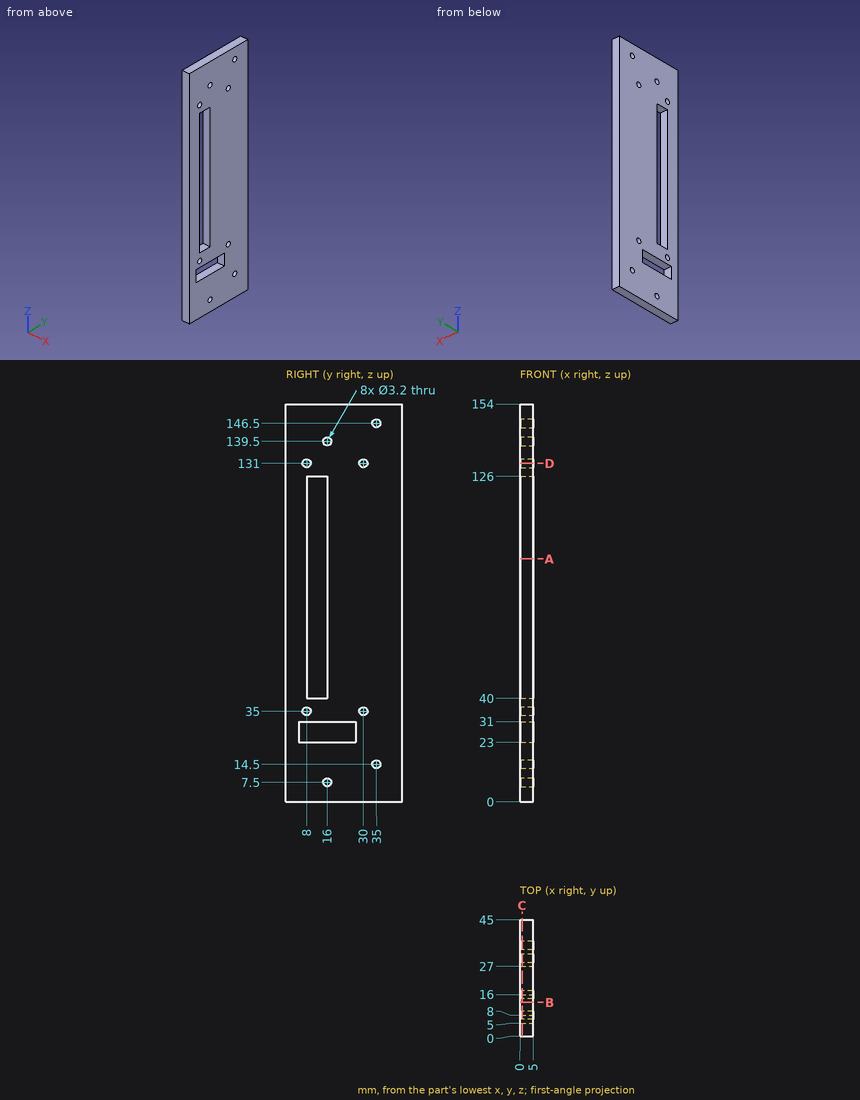
The figure shows three views and two pictorial views of one solid part (mm, origin at its lowest corner). Answer the questions. Round coordinates to 2 decimals unless told otherwise and drop trailing zeros. Order: outer loops, then holes, each group sorted by start corner. A loop starts at its lowest first (then second) coordinate and runs counter-clockwise, first axis right, second up. Notation, with made-up numbers: (49.25, -25) - (103.25, -25) arc R23 ccw to (103.25, 3) - close; hole circle Ø6 at (77, -20.75). An arc over 180 degrees is marked (long way). Write item = value, one per line. Start each with the question number.
1) Section A-A, the plane z = 94 is taken. Write down the section's boundary in (x, y), plus the area to 3 significant figures.
2) Section B-B, the plane y = 13 is taken. Write down the section's boundary in (x, z).
3) Section C-C, the plane x = 0.8 is taken. Count the separate pieces of the cut face and the enclosed holes in it, plus the area to 3 significant figures.
4) Section D-D, the plane z = 131 is taken. Write down the section's boundary in (x, y).
5) Straight lines are drawn through the part: L1, parallel to Z at x = 1.95, y = 12; L2, parallel to Z at x = 2.4, y = 30; L3, parallel to Y at x = 3.95, z = 35. For each, find the intervals that lie inside material, in ascending order.
Results list:
q1.outline = (0, 0) - (5, 0) - (5, 8) - (0, 8) - close; (0, 16) - (5, 16) - (5, 45) - (0, 45) - close
q1.area = 185 mm^2
q2.outline = (0, 0) - (5, 0) - (5, 23) - (0, 23) - close; (0, 31) - (5, 31) - (5, 40) - (0, 40) - close; (0, 126) - (5, 126) - (5, 154) - (0, 154) - close
q3.separate_pieces = 1
q3.enclosed_holes = 10
q3.area = 6,000 mm^2
q4.outline = (0, 0) - (5, 0) - (5, 6.4) - (0, 6.4) - close; (0, 9.6) - (5, 9.6) - (5, 28.4) - (0, 28.4) - close; (0, 31.6) - (5, 31.6) - (5, 45) - (0, 45) - close
q5.L1 = 0 to 23, 31 to 40, 126 to 154
q5.L2 = 0 to 33.4, 36.6 to 129.4, 132.6 to 154
q5.L3 = 0 to 6.4, 9.6 to 28.4, 31.6 to 45
